from build123d import *

# Parameters (mm, degrees)
SKETCH1_W           = 160
SKETCH1_H           = 80
BOSS_EXTRUDE1_DEPTH = 25
CUT_EXTRUDE1_START  = -80
CUT_EXTRUDE1_DEPTH  = 80


# Read off the part's stored shape, not the designer's step: Cut-Extrude1
with BuildPart() as part:
    # Sketch1 → Boss-Extrude1 (new body)
    with BuildSketch(Plane.XY):
        Rectangle(SKETCH1_W, SKETCH1_H)
    extrude(amount=BOSS_EXTRUDE1_DEPTH)

    # Cut-Extrude1 outline → Cut-Extrude1 (cut)
    with BuildSketch(Plane(origin=(0, 40, 0), x_dir=(1, 0, 0), z_dir=(0, 1, 0)).offset(CUT_EXTRUDE1_START)):
        Polygon((-80, 0), (-80, -10), (-69.65, -10), (-69.65, -5), (-72.7, -5), (-72.7, 0), align=None)
        Polygon((80, 0), (72.7, 0), (72.7, -5), (69.65, -5), (69.65, -10), (80, -10), align=None)
        Polygon((58.7, 0), (50.8, 0), (50.8, -5), (47.75, -5), (47.75, -10), (61.75, -10), (61.75, -5), (58.7, -5), align=None)
        Polygon((36.8, 0), (28.9, 0), (28.9, -5), (25.85, -5), (25.85, -10), (39.85, -10), (39.85, -5), (36.8, -5), align=None)
        Polygon((14.9, 0), (7, 0), (7, -5), (3.95, -5), (3.95, -10), (17.95, -10), (17.95, -5), (14.9, -5), align=None)
        Polygon((-7, 0), (-14.9, 0), (-14.9, -5), (-17.95, -5), (-17.95, -10), (-3.95, -10), (-3.95, -5), (-7, -5), align=None)
        Polygon((-28.9, 0), (-36.8, 0), (-36.8, -5), (-39.85, -5), (-39.85, -10), (-25.85, -10), (-25.85, -5), (-28.9, -5), align=None)
        Polygon((-50.8, 0), (-58.7, 0), (-58.7, -5), (-61.75, -5), (-61.75, -10), (-47.75, -10), (-47.75, -5), (-50.8, -5), align=None)
    extrude(amount=CUT_EXTRUDE1_DEPTH, mode=Mode.SUBTRACT)


solid = part.part
Design review of the part built by this model. Coordinates are the model's own, in mm. A direction names the side the tool comes from. Coordinates: 2 decimals unless noted, no trailing zeros. Loops run counter-clockwise (first coordinate to the right, second up) from the corner with the lowest first, then second, coordinate; pieces in that order, holes last. Notation, with made-up numbers: M 7,-32.5 L 48,-32.5 A23 cw 48,-1.5 Z; hole C 43,-3.5 d11. An arc over 180 degrees is marked long. Answer as CSV lines item,"result".
Item 1: For P1, Ø1.5, axis at y = 0, z = 2.5, coming from the -X side; P2, Ø1.5, axis at y = -12, z = 6.5, coming from the +X side; P3, Ø4, axis at y = 3.5, z = 3, coming from the +X side, all flat-tipped, find the tip position at first contact; note any pin that passes through.
Answer list:
P1,"x = -72.7"
P2,"x = 69.65"
P3,"x = 72.7"
Item 2: Machinability: for faces 1 (the face through (-33, -1, 10)), 2 (the face through (75, -1, 10)), 3 (the face through (36.8, -1, 3)), which of the approach directions +Z, -Z, +X, -X, +Y, -Y give a long, thin tool a straight path to every point of the face, cutting with its end or side? Answer none if there is none.
Answer list:
face 1,"+Y, -Y"
face 2,"+X, +Y, -Y"
face 3,"-Z, +Y, -Y"
Item 3: The part is to be moulded in two halves that separate along X. For faces 4 (the face through (72.7, -1, 2)), 5 (the face through (28.9, -1, 2)), 6 (the face through (-17.95, -1, 7)), 7 (the face through (-71, -1, 5)), say which applies: pulls with the +X half, pulls with the -X half, needs draft (parallel to the pull), parting line crosses it, or undercut.
Answer list:
face 4,"pulls with the +X half"
face 5,"undercut"
face 6,"undercut"
face 7,"needs draft"
Item 4: For probe 1 along Z at (x, y) = (5.5, 4); probe 2 along Z at (x, y) = (53, -34.5), list the stretches that pass through material, from the lowest coordinate up.
Answer list:
probe 1,"0 to 5, 10 to 25"
probe 2,"10 to 25"
Item 5: Add section A-A on x = -34. State the section outline as (y, z) points.
Answer list:
outline,"M -40,10 L 40,10 L 40,25 L -40,25 Z"
